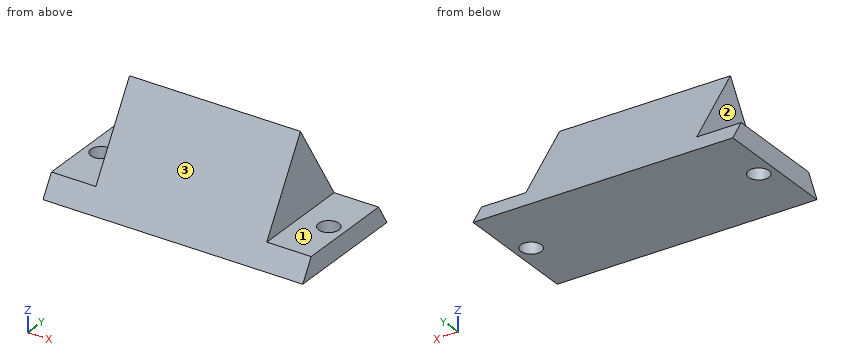
```python
from build123d import *

# Parameters (mm, degrees)
F0_W          = 38
F0_H          = 18.5
F0_R          = 1.5
F1_DEPTH      = 15
F3_DEPTH      = 38.001
F4_W          = 16.5
F4_H          = 12
F5_DEPTH      = 25
F5_DEPTH_BACK = 25


with BuildPart() as f1:
    # F0 (on Top) → F1 (new body)
    with BuildSketch(Plane.XY):
        Rectangle(F0_W, F0_H)
        with Locations((-16.65, 0)):
            Circle(F0_R, mode=Mode.SUBTRACT)
        with Locations((16.65, 0)):
            Circle(F0_R, mode=Mode.SUBTRACT)
    extrude(amount=F1_DEPTH)

    # F2 (on face) → F3 (cut, through all)
    with BuildSketch(Plane.YZ.offset(19)):
        Polygon((-9.25, 15), (-9.25, 0), (0, 15), align=None)
        Polygon((9.25, 15), (0, 15), (9.25, 0), align=None)
    extrude(amount=-F3_DEPTH, mode=Mode.SUBTRACT)

    # F4 (on Front) → F5 (cut, two sides)
    with BuildSketch(Plane.XZ) as f5_sk:
        with Locations((-20.75, 9)):
            Rectangle(F4_W, F4_H)
        with Locations((20.75, 9)):
            Rectangle(F4_W, F4_H)
    extrude(amount=F5_DEPTH, mode=Mode.SUBTRACT)
    extrude(f5_sk.sketch, amount=-F5_DEPTH_BACK, mode=Mode.SUBTRACT)


solid = f1.part
```
The model under review builds one solid part; all positions refer to its coordinate system, in mm. Face numbers are marked on the shaded views. A direction names the side the tool comes from. Round coordinates to 2 decimals unless told otherwise and drop trailing zeros. Write each loop counter-clockwise with the first axis right and the second up, starting at its lowest first coordinate (ties: lowest second). Pieces come first, ordered by that corner, then holes. Notation, with made-up numbers: (34, 71) - (70, 71) arc R22 ccw to (70, 81) - close; hole circle Ø11 at (-11.75, -35.75). An arc over 180 degrees is marked (long way). One line per question, with ' | ' between items.
Item 1: Add section A-A, the plane x = -16.65. Give the boundary of the cut face in (y, z), then the cut area to 4 significant figures.
Resolved:
outline: (-9.25, 0) - (-1.5, 0) - (-1.5, 3) - (-7.4, 3) - close; (1.5, 0) - (9.25, 0) - (7.4, 3) - (1.5, 3) - close | area: 40.95 mm2
Item 2: For the marked faces 1, 2 and 3, list the 3-axis set-ups (+Z, -Z, +X, -X, +Y, -Y) from which the entire face can be reached by the end or side of a thin tool; tool diameter is ignored.
Resolved:
face 1: +Z, +X, +Y, -Y | face 2: +Z, -X, +Y, -Y | face 3: +Z, +X, -X, -Y
Item 3: Add section B-B, the plane y = 4.75. Give the boundary of the cut face in (x, z), then the cut area to 3 significant figures.
Resolved:
outline: (-19, 0) - (19, 0) - (19, 3) - (12.5, 3) - (12.5, 7.3) - (-12.5, 7.3) - (-12.5, 3) - (-19, 3) - close | area: 221 mm2
Item 4: Add section D-D, the plane x = 16.5. Give the boundary of the cut face in (y, z).
Resolved:
outline: (-9.25, 0) - (-1.49, 0) - (-1.49, 3) - (-7.4, 3) - close; (1.49, 0) - (9.25, 0) - (7.4, 3) - (1.49, 3) - close
Item 5: To check wall thickness, follow probe 1 along Z at (x, y) = (-14.5, 5.25); probe 2 along Y at (x, z) = (-16.65, 1.5) (3 decimals); probe 3 along Z at (x, y) = (-5.5, -2.25). State the ranges of each line that lie inside material, in increasing order.
Resolved:
probe 1: z = 0 to 3 | probe 2: y = -8.325 to -1.5, 1.5 to 8.325 | probe 3: z = 0 to 11.35
Item 6: Add section C-C, the plane z = 9. Give the boundary of the cut face in (x, y), then the cut area to 3 significant figures.
Resolved:
outline: (-12.5, -3.7) - (12.5, -3.7) - (12.5, 3.7) - (-12.5, 3.7) - close | area: 185 mm2
Item 7: For P1, Ø5, axis at y = 0, z = 13, coming from the +X side; P2, Ø2, axis at x = -11, z = 9.5, coming from the +Y side; P3, Ø6, axis at y = -2.5, z = 8, coming from the -X side; P4, Ø3, axis at x = -12, y = 5, coming from the -Z side, all flat-tipped, find the tip position at first contact; note any pin that passes through.
Resolved:
P1: stops at x = 12.5 | P2: stops at y = 4.01 | P3: stops at x = -12.5 | P4: stops at z = 0
